from build123d import *

# Parameters (mm, degrees)
BOSS_EXTRUDE1_DEPTH = 5
SKETCH2_R           = 1.65
CUT_EXTRUDE1_DEPTH  = 5
SKETCH3_R           = 1.65
CUT_EXTRUDE2_DEPTH  = 19
CHAMFER1_SIZE       = 7
SKETCH4_R           = 3.15
CUT_EXTRUDE4_DEPTH  = 2


# Read off the part's stored shape, not the designer's step: Boss-Extrude1
with BuildPart() as part:
    # Boss-Extrude1 outline → Boss-Extrude1 (new body)
    with BuildSketch(Plane(origin=(0, 0, 0), x_dir=(1, 0, 0), z_dir=(0, 1, 0))):
        Polygon((18.5, 105), (3.5, 105), (3.5, 60), (-3.5, 60), (-3.5, 105), (-18.5, 105), (-18.5, 70), (-35, 51), (-55, 51), (-55, 0), (55, 0), (55, 51), (35, 51), (18.5, 70), align=None)
    extrude(amount=BOSS_EXTRUDE1_DEPTH)

    # Sketch2 → Cut-Extrude1 (cut)
    with BuildSketch(Plane(origin=(0, 0, 0), x_dir=(1, 0, 0), z_dir=(0, 1, 0))):
        with Locations(Location((-50, 5, 0), (0, 0, 90))):
            Circle(SKETCH2_R)
        with Locations(Location((-38, 5, 0), (0, 0, 90))):
            Circle(SKETCH2_R)
        with Locations(Location((50, 5, 0), (0, 0, 90))):
            Circle(SKETCH2_R)
        with Locations(Location((38, 5, 0), (0, 0, 90))):
            Circle(SKETCH2_R)
        with Locations(Location((-50, 46, 0), (0, 0, 90))):
            Circle(SKETCH2_R)
        with Locations(Location((-38, 46, 0), (0, 0, 90))):
            Circle(SKETCH2_R)
        with Locations(Location((50, 46, 0), (0, 0, 90))):
            Circle(SKETCH2_R)
        with Locations(Location((38, 46, 0), (0, 0, 90))):
            Circle(SKETCH2_R)
    extrude(amount=CUT_EXTRUDE1_DEPTH, mode=Mode.SUBTRACT)

    # Sketch3 → Cut-Extrude2 (cut)
    with BuildSketch(Plane(origin=(0, 0, 0), x_dir=(1, 0, 0), z_dir=(0, 1, 0))):
        with Locations(Location((-11, 88, 0), (0, 0, 90))):
            Circle(SKETCH3_R)
        with Locations(Location((11, 88, 0), (0, 0, 90))):
            Circle(SKETCH3_R)
        with Locations(Location((11, 98, 0), (0, 0, 90))):
            Circle(SKETCH3_R)
        with Locations(Location((-11, 98, 0), (0, 0, 90))):
            Circle(SKETCH3_R)
    extrude(amount=CUT_EXTRUDE2_DEPTH, mode=Mode.SUBTRACT)

    # Chamfer1
    chamfer1_edges = [part.edges().sort_by_distance(p)[0] for p in [
        (-3.5, 2.5, -105),
        (3.5, 2.5, -105),
    ]]
    chamfer(chamfer1_edges, length=CHAMFER1_SIZE)

    # Sketch4 → Cut-Extrude4 (cut)
    with BuildSketch(Plane(origin=(0, 0, 0), x_dir=(1, 0, 0), z_dir=(0, 1, 0))):
        with Locations(Location((-11, 98, 0), (0, 0, 270))):
            Circle(SKETCH4_R)
        with Locations(Location((11, 98, 0), (0, 0, 270))):
            Circle(SKETCH4_R)
        with Locations(Location((-11, 88, 0), (0, 0, 270))):
            Circle(SKETCH4_R)
        with Locations(Location((11, 88, 0), (0, 0, 270))):
            Circle(SKETCH4_R)
        with Locations(Location((-50, 46, 0), (0, 0, 270))):
            Circle(SKETCH4_R)
        with Locations(Location((-38, 46, 0), (0, 0, 270))):
            Circle(SKETCH4_R)
        with Locations(Location((38, 46, 0), (0, 0, 270))):
            Circle(SKETCH4_R)
        with Locations(Location((50, 46, 0), (0, 0, 270))):
            Circle(SKETCH4_R)
        with Locations(Location((38, 5, 0), (0, 0, 270))):
            Circle(SKETCH4_R)
        with Locations(Location((50, 5, 0), (0, 0, 270))):
            Circle(SKETCH4_R)
        with Locations(Location((-50, 5, 0), (0, 0, 270))):
            Circle(SKETCH4_R)
        with Locations(Location((-38, 5, 0), (0, 0, 270))):
            Circle(SKETCH4_R)
    extrude(amount=CUT_EXTRUDE4_DEPTH, mode=Mode.SUBTRACT)


solid = part.part
CAD build for the part. Positions are in the model's coordinates, mm. A direction names the side the tool comes from. Round coordinates to 2 decimals unless told otherwise and drop trailing zeros. Order: outer loops, then holes, each group sorted by start corner. A loop starts at its lowest first (then second) coordinate and runs counter-clockwise, first axis right, second up. Notation, with made-up numbers: (-24.75, -36.75) - (30.25, -36.75) arc R26 ccw to (30.25, -11.75) - close; hole circle Ø4 at (-2, 61). An arc over 180 degrees is marked (long way). Return JSON: item names as keys, results as strings.
(1) Tool access for faces 1 (the face through (3.5, 2, -79)), 2 (the face through (-26.635, 2.465, -60.633)), 3 (the face through (45, 2, -51)), 4 (the face through (36.6, 2, -44.6)), 5 (the face through (-39.115, 3.479, -44.784)): list every direction of +Z, -Z, +X, -X, +Y, -Y with a clear straight run to the whole face (end or side of a thin tool).
Answer key:
{"face 1": "-Z, +Y, -Y", "face 2": "-Z, -X, +Y, -Y", "face 3": "-Z, +X, +Y, -Y", "face 4": "-Y", "face 5": "+Y, -Y"}
(2) Wall check: probe 1 along X at (y, z) = (0.75, -88); probe 2 along X at (y, z) = (3.3, -88); probe 3 along Z at (x, y) = (50, 4.4). Give the ranges that are in metal, low to high. Write a range as from..to.
Answer key:
{"probe 1": "x = -18.5..-14.15, -7.85..-3.5, 3.5..7.85, 14.15..18.5", "probe 2": "x = -18.5..-12.65, -9.35..-3.5, 3.5..9.35, 12.65..18.5", "probe 3": "z = -51..-47.65, -44.35..-6.65, -3.35..0"}
(3) Pull direction X, two halves, no side cores. Call faces 6 (the face through (46.925, 0.986, -46.683)), 7 (the face through (-14, 2, -105)), 8 (the face through (-55, 2, -26)): +X half, -X half, draft (parallel to the pull), parting line (faces both ways), or undercut.
Answer key:
{"face 6": "undercut", "face 7": "draft", "face 8": "-X half"}
(4) Cut at A-A (x = -38). Give the cut face in (y, z).
Answer key:
{"outline": "(0, -51) - (5, -51) - (5, -47.65) - (2, -47.65) - (2, -49.15) - (0, -49.15) - close; (0, -42.85) - (2, -42.85) - (2, -44.35) - (5, -44.35) - (5, -6.65) - (2, -6.65) - (2, -8.15) - (0, -8.15) - close; (0, -1.85) - (2, -1.85) - (2, -3.35) - (5, -3.35) - (5, 0) - (0, 0) - close"}
(5) Cut at B-B (z = -88). Give the cut face in (x, y), then the cut area to 3 significant figures.
Answer key:
{"outline": "(-18.5, 0) - (-14.15, 0) - (-14.15, 2) - (-12.65, 2) - (-12.65, 5) - (-18.5, 5) - close; (-9.35, 2) - (-7.85, 2) - (-7.85, 0) - (-3.5, 0) - (-3.5, 5) - (-9.35, 5) - close; (3.5, 0) - (7.85, 0) - (7.85, 2) - (9.35, 2) - (9.35, 5) - (3.5, 5) - close; (12.65, 2) - (14.15, 2) - (14.15, 0) - (18.5, 0) - (18.5, 5) - (12.65, 5) - close", "area": "105 mm^2"}
(6) Cut at C-C (y = 3.5). State how many separate pieces and enclosed holes the cut face has, then the cut area to 3 significant figures.
Answer key:
{"separate pieces": "1", "enclosed holes": "12", "area": "7,450 mm^2"}
(7) Pin check, flat tips, straight feed: pin 1 Ø2.5 at (y, z) = (2.5, -72.5) entering from +X; pin 2 Ø1.9 at (x, z) = (51.5, -44.5) entering from -Y; pin 3 Ø1.5 at (x, y) = (6.5, 3.5) entering from -Z. Stop position of each tip, or through.
Answer key:
{"pin 1": "stops at x = 18.5", "pin 2": "stops at y = 2", "pin 3": "stops at z = -101.75"}
